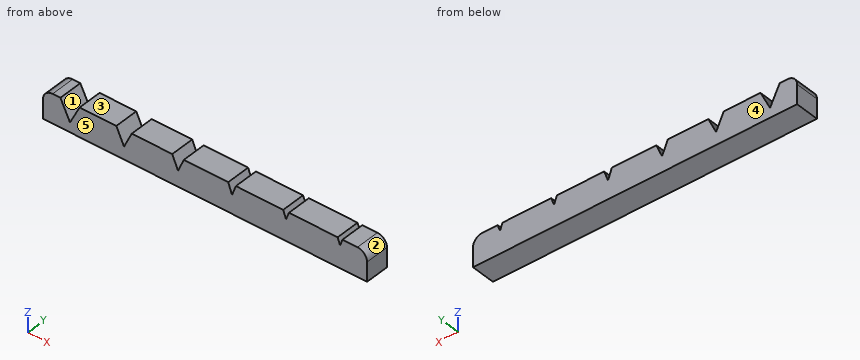
from build123d import *

# Parameters (mm, degrees)
F0_W     = 42.8244
F0_H     = 3.175
F1_DEPTH = 3.81
F3_DEPTH = 3.176
F4_R     = 1.27


with BuildPart() as f1:
    # F0 (on Top) → F1 (new body)
    with BuildSketch(Plane.XY):
        Rectangle(F0_W, F0_H)
    extrude(amount=-F1_DEPTH)

    # F2 (on face) → F3 (cut, through all)
    with BuildSketch(Plane.XZ.offset(1.5875)):
        Polygon((-16.571534, 0), (-19.111534, 0), (-17.841534, -2.54), align=None)
        Polygon((-9.688922, 0), (-11.720922, 0), (-10.704922, -2.159), align=None)
        Polygon((-2.806309, 0), (-4.330309, 0), (-3.568309, -1.778), align=None)
        Polygon((4.076304, 0), (3.060304, 0), (3.568304, -1.397), align=None)
        Polygon((10.704916, -1.016), (11.085916, 0), (10.323916, 0), align=None)
        Polygon((17.841529, -0.889), (18.159029, 0), (17.524029, 0), align=None)
    extrude(amount=-F3_DEPTH, mode=Mode.SUBTRACT)

    # F4
    f4_edges = [f1.edges().sort_by_distance(p)[0] for p in [
        (-21.4122, 0, 0),
        (21.4122, 0, 0),
    ]]
    fillet(f4_edges, radius=F4_R)


solid = f1.part
Geometry check sheet. Reference: the model listing, model coordinates, mm. Face numbers are marked on the shaded views. A direction names the side the tool comes from. Give positions to 0.01 mm unless a question says otherwise; leave off trailing zeros. Order: outer loops, then holes, each group sorted by start corner. A loop starts at its lowest first (then second) coordinate and runs counter-clockwise, first axis right, second up.
1. Access from +Z, -Z, +X, -X, +Y, -Y to the whole of each face (thin tool, end or side, straight path). Record for the marked faces 1 and 2.
Completed:
face 1: +Z, +Y, -Y
face 2: +Z, +X, +Y, -Y
2. Scan lines: line 1 (X direction, y = -0.3, z = -1.9); line 2 (Z direction, x = -10.5, y = 1.25); line 3 (Z direction, x = -17, y = -0.4). Record each from-to range of solid material in increasing order.
Completed:
line 1: x = -21.41 to -18.16, -17.52 to -10.83, -10.58 to 21.41
line 2: z = -3.81 to -1.72
line 3: z = -3.81 to -0.86
3. Sectioned sample at A-A (y = -0.95). Record the boundary of the cut face in (x, z).
Completed:
outline: (-21.41, -3.81) - (21.41, -3.81) - (21.41, -1.27) arc R1.27 ccw to (20.14, 0) - (18.16, 0) - (17.84, -0.89) - (17.52, 0) - (11.09, 0) - (10.7, -1.02) - (10.32, 0) - (4.08, 0) - (3.57, -1.4) - (3.06, 0) - (-2.81, 0) - (-3.57, -1.78) - (-4.33, 0) - (-9.69, 0) - (-10.7, -2.16) - (-11.72, 0) - (-16.57, 0) - (-17.84, -2.54) - (-19.11, 0) - (-20.14, 0) arc R1.27 ccw to (-21.41, -1.27) - close
4. Draft check along Y on the marked faces 3, 4 and 5. Enter one of: pulls with the +Y half, pulls with the -Y half, needs draft (parallel to the pull), parting line crosses it, or undercut.
Completed:
face 3: needs draft
face 4: pulls with the +Y half
face 5: pulls with the -Y half
